Work out the finished part from the listing and answer in its coordinate system (mm). A direction names the side the tool comes from. Give positions to 0.01 mm unless a question says otherwise; leave off trailing zeros. Loops run counter-clockwise (first coordinate to the right, second up) from the corner with the lowest first, then second, coordinate; pieces in that order, holes last. Notation, with made-up numbers: M 33,14 L 72,14 A26 cw 72,51 Z; hole C 57,6 d5. An arc over 180 degrees is marked long. Use a Markdown table: item, result.
Autodesk Inventor part; units mm, degrees
ref_plane "YZ Plane" through (0, 0, 0) normal (1, 0, 0) x (0, 1, 0)
ref_plane "XZ Plane" through (0, 0, 0) normal (0, 1, 0) x (-1, 0, 0)
ref_plane "XY Plane" through (0, 0, 0) normal (0, 0, 1) x (1, 0, 0)
sketch "Esquisse1" plane through (0, 0, 0) normal (1, 0, 0) x (0, 1, 0)
  line L0 (-2.5, 65) -> (2.5, 65)
  line L1 (2.5, 65) -> (2.5, -65)
  line L2 (2.5, -65) -> (-2.5, -65)
  line L3 (-2.5, -65) -> (-2.5, 65)
  line L4 (2.5, 65) -> (-2.5, -65)
  line L5 (2.5, -65) -> (-2.5, 65)
  point P0 (0, 0)
  point P1 (0, 0)
  point P2 (0, 0)
  dimension "d0" = 130
  dimension "d1" = 5
extrude "Extrusion1" add sketch "Esquisse1" along normal blind 5
sketch "Esquisse2" plane through (5, 0, 0) normal (1, 0, 0) x (0, 0, -1)
  line L0 (65, 2.5) -> (-65, 2.5)
  line L1 (-65, -2.5) -> (65, -2.5)
  line L2 (-30, 2.5) -> (-20, 2.5)
  line L3 (-20, 2.5) -> (-20, -2.5)
  line L4 (-20, -2.5) -> (-30, -2.5)
  line L5 (-30, -2.5) -> (-30, 2.5)
  line L6 (0, 13) -> (0, -16)
  line L7 (30, 2.5) -> (20, 2.5)
  line L8 (20, 2.5) -> (20, -2.5)
  line L9 (20, -2.5) -> (30, -2.5)
  line L10 (30, -2.5) -> (30, 2.5)
  point P0 (0, 0)
  point P1 (-20, 2.5)
  point P2 (30, -2.5)
  point P3 (30, 2.5)
  point P4 (20, 2.5)
  point P5 (20, -2.5)
  dimension "d4" = 10
  dimension "d5" = 20
extrude "Extrusion2" add sketch "Esquisse2" along normal blind 10 contours L10 L1 L8 L0 | L3 L1 L5 L0
sketch "Esquisse3" plane through (0, 2.5, 65) normal (0, 1, 0) x (1, 0, 0)
  line L0 (15, 45) -> (15, 35)
  line L1 (5, 45) -> (15, 45)
  line L2 (15, 35) -> (12, 35)
  line L3 (12, 35) -> (12, 45)
  line L4 (12, 45) -> (15, 45)
  line L5 (15, 45) -> (15, 35)
  line L6 (-9, 65) -> (24, 65)
  line L7 (15, 85) -> (15, 95)
  line L8 (15, 95) -> (12, 95)
  line L9 (12, 95) -> (12, 85)
  line L10 (12, 85) -> (15, 85)
  line L11 (15, 85) -> (15, 95)
  point P0 (0, 65)
extrude "Extrusion3" add sketch "Esquisse3" along normal blind 15
sketch "Esquisse4" plane through (15, 0, 0) normal (1, 0, 0) x (0, 0, -1)
  circle A0 centre (-25, 13.5) radius 1.75
  line L0 (0, 20) -> (0, -21)
  circle A1 centre (25, 13.5) radius 1.75
  line L1 (-30, 17.5) -> (-20, 17.5)
  line L2 (-20, -2.5) -> (-20, 17.5)
  point P0 (0, 0)
  dimension "d10" = 3.5
  dimension "d11" = 4
  dimension "d19" = 5
extrude "Extrusion4" cut sketch "Esquisse4" against normal blind 10
sketch "Esquisse6" plane through (0, -2.5, 65) normal (0, 0, 1) x (1, 0, 0)
  line L0 (0, 0) -> (5, 0)
  line L1 (5, 0) -> (5, -8)
  line L2 (5, -8) -> (-17, -8)
  line L3 (-17, -8) -> (5, 12)
  line L4 (5, 0) -> (5, 5)
  line L5 (5, 12) -> (5, 0)
  point P0 (0, 2.5)
extrude "Extrusion6" add sketch "Esquisse6" against normal blind 130
sketch "Esquisse8" plane through (12, 2.5, 20) normal (-1, 0, 0) x (0, 0, 1)
  line L0 (0, -5) -> (0, 15)
  line L1 (0, 0) -> (10, 0)
  line L2 (0, 15) -> (10, 15)
  line L3 (10, 15) -> (10, 0)
  line L4 (10, 0) -> (0, 0)
  line L5 (0, 0) -> (0, 15)
  line L6 (-50, -5) -> (-50, 15)
  line L7 (-40, 0) -> (-40, 15)
  line L8 (-50, 15) -> (-40, 15)
  line L9 (-40, 15) -> (-40, 0)
  line L10 (-40, 0) -> (-50, 0)
  line L11 (-50, 0) -> (-50, 15)
  circle A0 centre (5, 6) radius 1.75
  point P0 (-20, -2.5)
extrude "Extrusion7" cut sketch "Esquisse8" along normal blind 130 contours L0 L2 L3 L1 | L6 L8 L7 L10 | A0
sketch "Esquisse10" plane through (5, -2.5, -30) normal (0, -1, 0) x (1, 0, 0)
  line L0 (10, 0) -> (7, 0)
  line L1 (0, 10) -> (7, 10)
  line L2 (10, 0) -> (0, 0)
  line L3 (0, 0) -> (0, 10)
  line L4 (0, 10) -> (10, 10)
  line L5 (10, 10) -> (10, 0)
  line L6 (0, 60) -> (7, 60)
  line L7 (10, 50) -> (0, 50)
  line L8 (0, 50) -> (0, 60)
  line L9 (0, 60) -> (10, 60)
  line L10 (10, 60) -> (10, 50)
  point P0 (-5, 30)
extrude "Extrusion8" add sketch "Esquisse10" along normal blind 8
fillet "Congé5" radius 2 20 edges at (15, -10.5, -25) (15, -10.5, 25) (5, -10.5, -47.5) (5, -10.5, 0) (5, -10.5, 47.5) (10, -10.5, 20) (10, -10.5, 30) (10, -10.5, -20) (10, -10.5, -30) (-6, -10.5, -65) (5, -0.5, -65) (-6, -0.5, -65) (5, 9.5, -47.5) (5, 9.5, 0) (5, 9.5, 47.5) (5, -0.5, 65) (15, 3.5, 30) (15, 3.5, 20) (15, 3.5, -20) (15, 3.5, -30)
fillet "Congé6" radius 2 10 edges at (8, -10.5, 28) (4.4142, -9.9142, 29.4142) (5, -3, 30) (4.4142, -9.9142, -20.5858) (5, -3, -20) (4.4142, -9.9142, 20.5858) (5, -3, 20) (8, -10.5, -28) (4.4142, -9.9142, -29.4142) (5, -3, -30)
fillet "Congé7" radius 2 2 edges at (12, 2.5, -25) (12, 2.5, 25)
fillet "Congé8" radius 2 2 edges at (-2.7, 2.5, -25) (-2.7, 2.5, 25)
sketch "Esquisse12" plane through (-17, -10.5, 65) normal (0, 0, 1) x (1, 0, 0)
  line L0 (0, 0) -> (22, 20)
  line L1 (22, 20) -> (22, 0)
  line L2 (22, 13) -> (22, 2)
  line L3 (22, 0) -> (0, 0)
  point P0 (17, 10.5)
extrude "Extrusion9" cut sketch "Esquisse12" against normal blind 25
sketch "Esquisse13" plane through (3, -8.5, -65) normal (0, 0, -1) x (-1, 0, 0)
  line L0 (0, -2) -> (20, -2)
  line L1 (20, -2) -> (-2, 18)
  line L2 (-2, 18) -> (-2, -2)
  line L3 (-2, 11) -> (-2, 0)
  line L4 (-2, -2) -> (20, -2)
  point P0 (3, 8.5)
extrude "Extrusion10" cut sketch "Esquisse13" against normal blind 25
properties part number "pare-chocs_Impression 3D"
(1) A cutting plane is placed at B-B (y = -7). Write down the section's boundary in (x, z), and give its area (3 significant figures).
Entries:
| item | result |
|---|---|
| outline | M -13.15,-40 L 5,-40 L 5,-32 A2 cw 7,-30 L 13,-30 A2 ccw 15,-28 L 15,-22 A2 ccw 13,-20 L 7,-20 A2 cw 5,-18 L 5,18 A2 cw 7,20 L 13,20 A2 ccw 15,22 L 15,28 A2 ccw 13,30 L 7,30 A2 cw 5,32 L 5,40 L -13.15,40 Z |
| area | 1,650 mm² |
(2) A cutting plane is placed at D-D (x = -1). Write down the section's boundary in (y, z), and give its area (3 significant figures).
Entries:
| item | result |
|---|---|
| outline | M -10.5,-40 L 4.05,-40 L 4.05,-30 L 2.5,-30 L 2.5,-20 L 4.05,-20 L 4.05,20 L 2.5,20 L 2.5,30 L 4.05,30 L 4.05,40 L -10.5,40 Z |
| area | 1,130 mm² |
(3) Consider probe 1 along Y at (x, z) = (13, 25); probe 2 along Z at (x, y) = (13, 14.5); probe 3 along Y at (x, z) = (13.7, 25). Determine where each line is inside the solid, lowest interval first. Write a range as [from, to].
Entries:
| item | result |
|---|---|
| probe 1 | y = [-10.5, 11.75], [15.25, 17.5] |
| probe 2 | z = [-30, -26.44], [-23.56, -20], [20, 23.56], [26.44, 30] |
| probe 3 | y = [-10.37, 11.75], [15.25, 17.5] |
(4) A cutting plane is placed at C-C (z = 3). Write down the section's boundary in (x, y).
Entries:
| item | result |
|---|---|
| outline | M -17,-10.5 L 3,-10.5 A2 ccw 5,-8.5 L 5,4.98 A2 ccw 1.65,6.46 Z |
(5) Which of the six approach directions +Z, -Z, +X, -X, +Y, -Y give full straight-line access (tool end or side, diameter ignored) to faces 5 (the cylindrical face through (4.43, -9.9, -0.31)), 6 (the flat face through (2, 4, 20)), 7 (the cylindrical face through (5.6, -2.92, -19.43)), 8 (the cylindrical face through (9.04, -9.9, -29.43)), 9 (the flat face through (12, 11, -25))?
Entries:
| item | result |
|---|---|
| face 5 | +X, -Y |
| face 6 | -X, +Y |
| face 7 | +X, +Y, -Y |
| face 8 | -Z, +X, -Y |
| face 9 | +Z, -Z, -X, +Y |
(6) A cutting plane is placed at A-A (z = -25). Write down the section's boundary in (x, y).
Entries:
| item | result |
|---|---|
| outline | M -17,-10.5 L 13,-10.5 A2 ccw 15,-8.5 L 15,11.75 L 12,11.75 L 12,4.5 A2 cw 10,2.5 L -1.93,2.5 A2 ccw -3.27,1.98 Z; M 12,15.25 L 15,15.25 L 15,17.5 L 12,17.5 Z |
(7) Given P1, Ø3, axis at y = 8, z = -13, coming from the -X side; P2, Ø11, axis at y = 11, z = 25, coming from the -X side; P3, Ø3, axis at x = 9, y = 11, coming from the +Z side; P4, Ø9.5, axis at x = 6, z = -25, coming from the +Y side, each flat-ended and moving along its own axis, determine where each tip first touches the part or whether it passes through.
Entries:
| item | result |
|---|---|
| P1 | stops at x = 1.7 |
| P2 | stops at x = 12 |
| P3 | passes through |
| P4 | stops at y = 2.65 |
(8) The mould has two halves that part along Z. Classify faces 1 (the flat face through (10, -1, -30)), 2 (the cylindrical face through (9.18, -9.9, 29.43)), 3 (the cylindrical face through (4.43, -9.9, -35.42)), 4 (the cylindrical face through (5.57, -2.92, 19.4)): released by +Z, released by -Z, zero draft, split by the parting line, or undercut.
Entries:
| item | result |
|---|---|
| face 1 | released by -Z |
| face 2 | released by +Z |
| face 3 | zero draft |
| face 4 | undercut |
